Design review of the part built by this model. Coordinates are the model's own, in mm. Face numbers are marked on the shaded views. A direction names the side the tool comes from. Give positions to 0.01 mm unless a question says otherwise; leave off trailing zeros. Order: outer loops, then holes, each group sorted by start corner. A loop starts at its lowest first (then second) coordinate and runs counter-clockwise, first axis right, second up. Notation, with made-up numbers: M 73.5,3.25 L 93.5,3.25 A21 ccw 93.5,39.25 Z; hole C 10.25,58.25 d9. An arc over 180 degrees is marked long. Put each result on its own line as item: value. Start each with the question number.
from build123d import *

# Parameters (mm, degrees)
F0_R     = 6.75
F1_DEPTH = 3.6
F2_DEPTH = 1
F3_R     = 1
F4_DEPTH = 25
F6_DEPTH = 10
F8_R     = 3.5
F9_DEPTH = 10


with BuildPart() as f1:
    # F0 (on Top) → F1 (new body)
    with BuildSketch(Plane.XY):
        Circle(F0_R)
        Polygon((-4.6808759634, 2.7464037483), (0.0380174333, 5.4269593704), (4.7188933967, 2.6805556222), (4.6808759634, -2.7464037483), (-0.0380174333, -5.4269593704), (-4.7188933967, -2.6805556222), align=None, mode=Mode.SUBTRACT)
    extrude(amount=F1_DEPTH)

    # F0 (on Top) → F2 (join)
    with BuildSketch(Plane.XY):
        Polygon((4.7188933967, 2.6805556222), (0.0380174333, 5.4269593704), (-4.6808759634, 2.7464037483), (-4.7188933967, -2.6805556222), (-0.0380174333, -5.4269593704), (4.6808759634, -2.7464037483), align=None)
    extrude(amount=F2_DEPTH)

    # F3 (on face) → F4 (cut)
    with BuildSketch(Plane.XY.offset(1)):
        Circle(F3_R)
    extrude(amount=-F4_DEPTH, mode=Mode.SUBTRACT)

    # F5 (on face) → F6 (join)
    with BuildSketch(Plane.XY):
        with BuildLine():
            ThreePointArc((0.3, -0.9539392014), (0, -1), (-0.3, -0.9539392014))
            add(Edge.make_bspline(
                [(-0.3, -0.9539392014), (-0.2571564854, -1.7815360064), (-0.0005705868, -3.4185465418), (0.2582976589, -1.7813709101), (0.3, -0.9539392014)],
                knots=[0, 0, 0, 0, 0.5, 1, 1, 1, 1], degree=3))
        make_face()
    extrude(amount=-F6_DEPTH)

    # F8 (on face) → F9 (join)
    with BuildSketch(Plane(origin=(0, 0, 0), x_dir=(1, 0, 0), z_dir=(0, 0, -1))):
        Circle(F8_R)
        with BuildLine():
            ThreePointArc((0.3, 0.9539392014), (0.8062257748, 0.5916079783), (1, 0))
            ThreePointArc((1, 0), (-0.5916079783, -0.8062257748), (-0.3, 0.9539392014))
            add(Edge.make_bspline(
                [(-0.3, 0.9539392014), (-0.2571564854, 1.7815360064), (-0.0005705868, 3.4185465418), (0.2582976589, 1.7813709101), (0.3, 0.9539392014)],
                knots=[0, 0, 0, 0, 0.5, 1, 1, 1, 1], degree=3))
        make_face(mode=Mode.SUBTRACT)
    extrude(amount=F9_DEPTH)


solid = f1.part
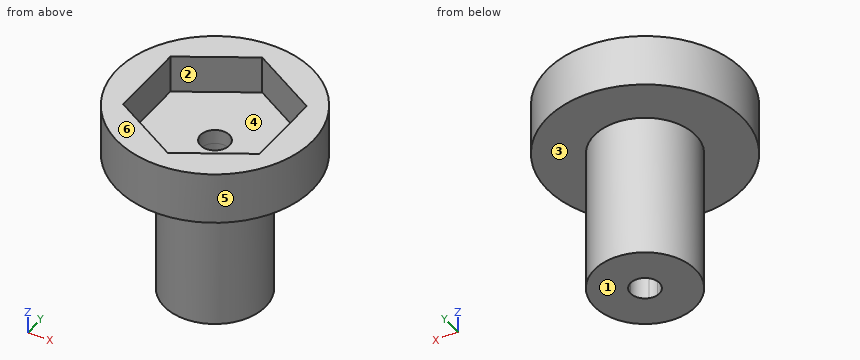
1. Consider section D-D on x = -4. Give the boundary of the cut face in (y, z), then the cut area to 3 significant figures.
2. Machinability: for the marked faces 1, 2 and 3, which of the approach directions +Z, -Z, +X, -X, +Y, -Y give a long, thin tool a straight path to every point of the face, cutting with its end or side? Answer none if there is none.
3. Insertion check: pin 1 (2 mm diameter, centred on y = 1, z = -5.5, fed in from +X); pin 2 (2 mm diameter, centred on y = -0.5, z = -4.5, fed in from -X); pin 3 (3 mm diameter, centred on y = -3, z = -1, fed in from +X). Each pin has a flat end and moves straight along its axis. Give the tip position at first contact, or say it passes through.
4. Consider section C-C on y = -0.5. Give the boundary of the cut face in (x, z), then the cut area to 3 significant figures.
5. Consider section B-B on x = 0.5. Give the boundary of the cut face in (y, z).
6. The part is to be moulded in two halves that separate along X. For the marked faces 4, 5 and 6, say which applies: +X half, -X half, draft (parallel to the pull), parting line (faces both ways), or undercut.
7. To check wall thickness, follow probe 1 along Y at (x, z) = (0, 0.4); probe 2 along Y at (x, z) = (0, -3.75); probe 3 along Z at (x, y) = (-3, -5.5). State the ranges of each line that lie inside material, in increasing order.
8. Consider section A-A on z = 2.75. Give the boundary of the cut face in (x, y), then the cut area to 3 significant figures.
Returned:
1. outline: M -5.44,0 L 5.44,0 L 5.44,3.6 L 3.13,3.6 L 3.13,1 L -3.1,1 L -3.1,3.6 L -5.44,3.6 Z
1. area: 22.9 mm2
2. face 1: -Z, +X, -X, +Y, -Y
2. face 2: +Z
2. face 3: -Z
3. pin 1: stops at x = 3.5
3. pin 2: stops at x = -3.5
3. pin 3: stops at x = 6.48
4. outline: M -6.73,0 L -3.46,0 L -3.46,-10 L -0.87,-10 L -0.87,1 L -4.7,1 L -4.7,3.6 L -6.73,3.6 Z; M 0.87,-10 L 3.46,-10 L 3.46,0 L 6.73,0 L 6.73,3.6 L 4.7,3.6 L 4.7,1 L 0.87,1 Z
4. area: 74.3 mm2
5. outline: M -6.73,0 L -3.46,0 L -3.46,-10 L -0.87,-10 L -0.87,1 L -5.12,1 L -5.12,3.6 L -6.73,3.6 Z; M 0.87,-10 L 3.46,-10 L 3.46,0 L 6.73,0 L 6.73,3.6 L 5.16,3.6 L 5.16,1 L 0.87,1 Z
6. face 4: undercut
6. face 5: parting line
6. face 6: draft
7. probe 1: y = -6.75 to -1, 1 to 6.75
7. probe 2: y = -3.5 to -1, 1 to 3.5
7. probe 3: z = 0 to 3.6
8. outline: C 0,0 d13.5; hole M -4.72,-2.68 L -0.04,-5.43 L 4.68,-2.75 L 4.72,2.68 L 0.04,5.43 L -4.68,2.75 Z
8. area: 66.6 mm2
